For this review, take the finished solid that the model builds, in its own axes (mm). A direction names the side the tool comes from. Give positions to 0.01 mm unless a question says otherwise; leave off trailing zeros. Order: outer loops, then holes, each group sorted by start corner. A loop starts at its lowest first (then second) coordinate and runs counter-clockwise, first axis right, second up. Notation, with made-up numbers: M 34.5,49.25 L 83.5,49.25 A34 cw 83.5,84.25 Z; hole C 30.5,70.5 d7. An arc over 180 degrees is marked long. Use CSV: the item, a comma, the result in double quotes. Start each with the question number.
(1) Consider section D-D (y = 9.5). Write out the cut boundary in (x, z), and give its area (3 significant figures).
(2) Consider section C-C (x = 29). Write out the cut boundary in (y, z), and give its area (3 significant figures).
(3) Consider section B-B (x = 20.5). Write out the cut boundary in (y, z).
(4) Clearance check with flat-ended pins moving along their axes: P1, Ø1.5, axis at y = -17.5, z = -13, coming from the -X side; P2, Ø13.5, axis at x = 21, y = 19.05, coming from the -Z side; P3, Ø7.5, axis at x = -30.67, y = 7.52, coming from the +Z side. State where each tip first meets the part, or that it passes through.
(5) Tool access review of faces 4 (the face through (-8.45, -17.64, -9.61)), 5 (the face through (37.993, 0.616, 0.986)), 6 (the face through (21, 19, 2)): name each direction out of +Z, -Z, +X, -X, +Y, -Y from which nothing blocks a thin tool from reaching the whole face with its end or side.
(6) Draft analysis for pull direction X (two halves, no side actions). For faces 1 (the face through (0, -28, 1)), 2 (the face through (-37.993, -0.616, 0.986)), 3 (the face through (21, -19, 2)), state which applies: pulls with the +X half, pulls with the -X half, needs draft (parallel to the pull), parting line crosses it, or undercut.
(7) Wall thickness on L1, parallel to Y at x = 21, z = 2.2; L2, parallel to X at y = -16, z = 0.75; L3, parallel to Z at x = -6, y = -1.5: over which ranges is each line inside the solid? List them lowest first. Write a range as from..to.
(8) Consider section A-A (y = 16). Write out the cut boundary in (x, z), and give its area (3 significant figures).
```python
from build123d import *

# Parameters (mm, degrees)
EXTRUDE_2_DEPTH           = 2
HOLE_WIZARD_0_D           = 2.8
HOLE_WIZARD_0_DEPTH       = 10.1
HOLE_WIZARD_0_CSINK_D     = 4.8
HOLE_WIZARD_0_CSINK_ANGLE = 90
HOLE_WIZARD_0_TIP         = 0.841204867
SKETCH_7_R                = 5.75
SKETCH_7_R_2              = 4.25
EXTRUDE_1_DEPTH           = 0.5
EXTRUDE_2_2_DEPTH         = 21.5
CHAMFER_1_SIZE            = 1.5


with BuildPart() as part:
    # 草图3 → Extrude 2 (new body)
    with BuildSketch(Plane.XY):
        with BuildLine():
            Line((10, -28), (-10, -28))
            ThreePointArc((-10, -28), (-38, 0), (-10, 28))
            Line((-10, 28), (10, 28))
            ThreePointArc((10, 28), (38, 0), (10, -28))
        make_face()
    extrude(amount=EXTRUDE_2_DEPTH)

    # 打孔尺寸(%根据十字)槽沉头自攻螺钉的类型0
    with Locations(Plane.XY.offset(2)):
        with Locations((-29, 16), (-29, -16), (29, 16), (29, -16)):
            CounterSinkHole(HOLE_WIZARD_0_D / 2, HOLE_WIZARD_0_CSINK_D / 2, depth=HOLE_WIZARD_0_DEPTH, counter_sink_angle=HOLE_WIZARD_0_CSINK_ANGLE)
            with Locations((0, 0, -(HOLE_WIZARD_0_DEPTH + HOLE_WIZARD_0_TIP / 2))):  # 118° drill point
                Cone(0, HOLE_WIZARD_0_D / 2, HOLE_WIZARD_0_TIP, mode=Mode.SUBTRACT)

    # 草图7 → 拉伸-薄壁1 (add)
    # profile 1 of 4: a face of its own
    with BuildSketch(Plane.XY.offset(2)):
        with Locations((-30.673237657, 7.524443153)):
            Circle(SKETCH_7_R)
        with Locations((-30.673237657, 7.524443153)):
            Circle(SKETCH_7_R_2, mode=Mode.SUBTRACT)
    # profile 2 of 4: a face of its own
    with BuildSketch(Plane.XY.offset(2)):
        with Locations((-30.673237657, -7.524443153)):
            Circle(SKETCH_7_R)
        with Locations((-30.673237657, -7.524443153)):
            Circle(SKETCH_7_R_2, mode=Mode.SUBTRACT)
    # profile 3 of 4: a face of its own
    with BuildSketch(Plane.XY.offset(2)):
        with Locations((21, -19.052558883)):
            Circle(SKETCH_7_R)
        with Locations((21, -19.052558883)):
            Circle(SKETCH_7_R_2, mode=Mode.SUBTRACT)
    # profile 4 of 4: a face of its own
    with BuildSketch(Plane.XY.offset(2)):
        with Locations((21, 19.052558883)):
            Circle(SKETCH_7_R)
        with Locations((21, 19.052558883)):
            Circle(SKETCH_7_R_2, mode=Mode.SUBTRACT)
    extrude(amount=EXTRUDE_1_DEPTH)

    # 草图10 → Extrude 2 2 (add)
    with BuildSketch(Plane.XY.offset(2)):
        with BuildLine():
            ThreePointArc((-24.214911699, -8.37772555), (-17.550101998, -14.671263061), (-8.554999344, -16.436604671))
            Line((-8.554999344, -16.436604671), (-8.336059851, -18.926999318))
            ThreePointArc((-8.336059851, -18.926999318), (-18.694056847, -16.894181707), (-26.368686199, -9.647077906))
            Line((-26.368686199, -9.647077906), (-24.214911699, -8.37772555))
        make_face()
    extrude(amount=-EXTRUDE_2_2_DEPTH)

    # 倒角1
    chamfer_1_edges = [part.edges().sort_by_distance(p)[0] for p in [
        (-17.550101998, -14.671263061, 0),
        (-18.694056847, -16.894181707, 0),
    ]]
    chamfer(chamfer_1_edges, length=CHAMFER_1_SIZE)


solid = part.part
```
Check result:
1,outline,"M -36.34,0 L 36.34,0 L 36.34,2 L -25.27,2 L -25.27,2.5 L -26.91,2.5 L -26.91,2 L -34.44,2 L -34.44,2.5 L -36.07,2.5 L -36.07,2 L -36.34,2 Z"
1,area,"147 mm^2"
2,outline,"M -20.57,0 L -17.4,0 L -17.4,1 L -18.4,2 L -20.57,2 Z; M -14.6,0 L 14.6,0 L 14.6,1 L 13.6,2 L -13.6,2 L -14.6,1 Z; M 17.4,0 L 20.57,0 L 20.57,2 L 18.4,2 L 17.4,1 Z"
2,area,"69.1 mm^2"
3,outline,"M -25.96,0 L 25.96,0 L 25.96,2 L 24.78,2 L 24.78,2.5 L 23.27,2.5 L 23.27,2 L 14.83,2 L 14.83,2.5 L 13.32,2.5 L 13.32,2 L -13.32,2 L -13.32,2.5 L -14.83,2.5 L -14.83,2 L -23.27,2 L -23.27,2.5 L -24.78,2.5 L -24.78,2 L -25.96,2 Z"
4,P1,"stops at x = -18.97"
4,P2,"stops at z = 0"
4,P3,"stops at z = 2"
5,face 4,"-Z, +X, +Y"
5,face 5,"+Z, -Z, +X"
5,face 6,"+Z"
6,face 1,"needs draft"
6,face 2,"pulls with the -X half"
6,face 3,"undercut"
7,L1,"y = -24.8..-23.3, -14.8..-13.3, 13.3..14.8, 23.3..24.8"
7,L2,"x = -32.98..-30.4, -27.6..27.6, 30.4..32.98"
7,L3,"z = 0..2"
8,outline,"M -32.98,0 L -30.4,0 L -30.4,1 L -31.4,2 L -32.98,2 Z; M -27.6,0 L 27.6,0 L 27.6,1 L 26.6,2 L 25.87,2 L 25.87,2.5 L 23.96,2.5 L 23.96,2 L 18.04,2 L 18.04,2.5 L 16.13,2.5 L 16.13,2 L -26.6,2 L -27.6,1 Z; M 30.4,0 L 32.98,0 L 32.98,2 L 31.4,2 L 30.4,1 Z"
8,area,"121 mm^2"
